from build123d import *

# Parameters (mm, degrees)
SKETCH1_R               = 11.7
BOSS_EXTRUDE1_DEPTH     = 35
SKETCH2_R               = 10
BOSS_EXTRUDE3_DEPTH     = 51.8
SKETCH3_R               = 3
CUT_EXTRUDE1_DEPTH      = 1
CUT_EXTRUDE1_DEPTH_BACK = 57.8
SKETCH6_W               = 28.4
SKETCH6_H               = 118.8
CUT_EXTRUDE3_DEPTH      = 36
SKETCH8_R               = 10
SKETCH8_R_2             = 3
CUT_EXTRUDE4_DEPTH      = 5
SKETCH7_R               = 4
SKETCH7_R_2             = 3
CUT_EXTRUDE5_DEPTH      = 5
FILLET1_R               = 10


with BuildPart() as part:
    # Sketch1 → Boss-Extrude1 (new body)
    with BuildSketch(Plane(origin=(0, 0, 0), x_dir=(0, 0, -1), z_dir=(1, 0, 0))):
        Polygon((-28.4, -59.4), (-23.4, -59.4), (-23.4, -14.4), (23.4, -14.4), (23.4, -59.4), (28.4, -59.4), (28.4, 59.4), (-28.4, 59.4), align=None)
        with Locations((0, 24)):
            Circle(SKETCH1_R, mode=Mode.SUBTRACT)
    extrude(amount=BOSS_EXTRUDE1_DEPTH)

    # Sketch2 → Boss-Extrude3 (add)
    with BuildSketch(Plane.XY.offset(28.4)):
        with Locations((17.5, -34.4)):
            Circle(SKETCH2_R)
        with BuildLine():
            Line((0, -24.717541634), (0, -13.4))
            Line((0, -13.4), (35, -13.4))
            Line((35, -13.4), (35, -24.717541634))
            ThreePointArc((35, -24.717541634), (17.5, -14.4), (0, -24.717541634))
        make_face()
    extrude(amount=-BOSS_EXTRUDE3_DEPTH)

    # Sketch3 → Cut-Extrude1 (cut, two sides)
    with BuildSketch(Plane.XY.offset(28.4)) as cut_extrude1_sk:
        with Locations((10.25, 49.4)):
            Circle(SKETCH3_R)
        with Locations((17.5, -34.4)):
            Circle(SKETCH3_R)
        with Locations((10.25, 2.3)):
            Circle(SKETCH3_R)
        with Locations((24.75, 2.3)):
            Circle(SKETCH3_R)
        with Locations((24.75, 49.4)):
            Circle(SKETCH3_R)
    extrude(amount=CUT_EXTRUDE1_DEPTH, mode=Mode.SUBTRACT)
    extrude(cut_extrude1_sk.sketch, amount=-CUT_EXTRUDE1_DEPTH_BACK, mode=Mode.SUBTRACT)

    # Sketch6 → Cut-Extrude3 (cut, through all)
    with BuildSketch(Plane(origin=(35, 0, 0), x_dir=(0, 0, -1), z_dir=(1, 0, 0))):
        with Locations((14.2, 0)):
            Rectangle(SKETCH6_W, SKETCH6_H)
    extrude(amount=-CUT_EXTRUDE3_DEPTH, mode=Mode.SUBTRACT)

    # Sketch8 → Cut-Extrude4 (cut)
    with BuildSketch(Plane(origin=(0, 0, 0), x_dir=(-1, 0, 0), z_dir=(0, 0, -1))):
        with Locations((-17.5, -34.4)):
            Circle(SKETCH8_R)
        with Locations((-17.5, -34.4)):
            Circle(SKETCH8_R_2, mode=Mode.SUBTRACT)
    extrude(amount=-CUT_EXTRUDE4_DEPTH, mode=Mode.SUBTRACT)

    # Sketch7 → Cut-Extrude5 (cut)
    with BuildSketch(Plane(origin=(0, 0, 0), x_dir=(-1, 0, 0), z_dir=(0, 0, -1))):
        with Locations((-24.75, 49.4)):
            Circle(SKETCH7_R)
        with Locations((-24.75, 49.4)):
            Circle(SKETCH7_R_2, mode=Mode.SUBTRACT)
        with Locations((-10.25, 49.4)):
            Circle(SKETCH7_R)
        with Locations((-10.25, 49.4)):
            Circle(SKETCH7_R_2, mode=Mode.SUBTRACT)
        with Locations((-24.75, 2.3)):
            Circle(SKETCH7_R)
        with Locations((-24.75, 2.3)):
            Circle(SKETCH7_R_2, mode=Mode.SUBTRACT)
        with Locations((-10.25, 2.3)):
            Circle(SKETCH7_R)
        with Locations((-10.25, 2.3)):
            Circle(SKETCH7_R_2, mode=Mode.SUBTRACT)
    extrude(amount=-CUT_EXTRUDE5_DEPTH, mode=Mode.SUBTRACT)

    # Fillet1
    fillet1_edges = [part.edges().sort_by_distance(p)[0] for p in [
        (0, 59.4, 14.2),
        (35, 59.4, 14.2),
    ]]
    fillet(fillet1_edges, radius=FILLET1_R)


solid = part.part
Source: CAD feature listing. Evaluate the final solid. Frame: model axes, mm. A direction names the side the tool comes from. Give positions to 0.01 mm unless a question says otherwise; leave off trailing zeros. Write each loop counter-clockwise with the first axis right and the second up, starting at its lowest first coordinate (ties: lowest second). Pieces come first, ordered by that corner, then holes. Notation, with made-up numbers: M -22.75,11 L 36.25,11 A25 ccw 36.25,35 Z; hole C 69,1.5 d4. An arc over 180 degrees is marked long. Return JSON: item names as keys, results as strings. Group by question number.
1) Draft query along Y for faces 3 (the face through (11.117, 45.495, 2.465)), 4 (the face through (3.01, 56.55, 14.4)), 5 (the face through (18, 47, 0)), 6 (the face through (17, -59.4, 26)). Return one class per face: released by +Y, released by -Y, zero draft, split by the parting line, or undercut.
2) Ray query, L1, parallel to X at y = 2.3, z = 13.75; L2, parallel to Y at x = 10.25, z = 1.3; L3, parallel to Y at x = 10.25, z = 12.75. Return the intervals inside material, ascending.
3) Cut plane D-D, the plane y = -34.4. Output: boundary loops of the cut face in (x, z).
4) Cut plane B-B, the plane x = 17.5. Output: boundary loops of the cut face in (y, z), then the cut area to 3 significant figures.
5) Cut plane A-A, the plane y = 2.3. Output: boundary loops of the cut face in (x, z), then the cut area to 3 significant figures.
6) Cut plane C-C, the plane x = 23. Output: boundary loops of the cut face in (y, z).
7) First-contact query: pin 1 Ø7 at (x, y) = (10.25, 49.4) entering from -Z; pin 2 Ø4 at (x, z) = (31, 16.5) entering from -Y; pin 3 Ø4 at (x, y) = (16.5, 25.5) entering from -Z. Flat tips, straight axial feed; report the tip coordinate or a pass-through.
8) Set-up query: faces 1 (the face through (22.88, -25.97, 14.33)), 2 (the face through (17.255, 24.257, 11.697)). Return all of +Z, -Z, +X, -X, +Y, -Y with unobstructed straight access to the full face (end or side cutting, diameter ignored); none if empty.
Data:
{
 "1": {"face 3": "undercut", "face 4": "released by +Y", "face 5": "zero draft", "face 6": "released by -Y"},
 "2": {"L1": "x = 0 to 7.25, 13.25 to 21.75, 27.75 to 35", "L2": "y = -15.76 to -1.7, 6.3 to 12.37, 35.63 to 45.4, 53.4 to 59.4", "L3": "y = -41.29 to -27.51, -15.76 to -0.7, 5.3 to 46.4, 52.4 to 59.4"},
 "3": {"outline": "M 0,23.4 L 7.5,23.4 L 7.5,5 L 14.5,5 L 14.5,28.4 L 0,28.4 Z; M 20.5,5 L 27.5,5 L 27.5,23.4 L 35,23.4 L 35,28.4 L 20.5,28.4 Z"},
 "4": {"outline": "M -59.4,23.4 L -44.4,23.4 L -44.4,5 L -37.4,5 L -37.4,28.4 L -59.4,28.4 Z; M -31.4,5 L -24.4,5 L -24.4,23.4 L -14.4,23.4 L -14.4,0 L 12.3,0 A11.7 cw 35.7,0 L 59.4,0 L 59.4,28.4 L -31.4,28.4 Z", "area": "2,330 mm²"},
 "5": {"outline": "M 0,0 L 6.25,0 L 6.25,5 L 7.25,5 L 7.25,28.4 L 0,28.4 Z; M 13.25,5 L 14.25,5 L 14.25,0 L 20.75,0 L 20.75,5 L 21.75,5 L 21.75,28.4 L 13.25,28.4 Z; M 27.75,5 L 28.75,5 L 28.75,0 L 35,0 L 35,28.4 L 27.75,28.4 Z", "area": "633 mm²"},
 "6": {"outline": "M -59.4,23.4 L -42.75,23.4 L -42.75,5 L -26.05,5 L -26.05,23.4 L -15.17,23.4 L -15.17,0 L -1.3,0 L -1.3,5 L -0.14,5 L -0.14,28.4 L -59.4,28.4 Z; M 4.74,5 L 5.9,5 L 5.9,0 L 12.3,0 A11.7 cw 35.7,0 L 45.8,0 L 45.8,5 L 46.96,5 L 46.96,28.4 L 4.74,28.4 Z; M 51.84,5 L 53,5 L 53,0 L 59.4,0 L 59.4,28.4 L 51.84,28.4 Z"},
 "7": {"pin 1": "stops at z = 5", "pin 2": "stops at y = -21.76", "pin 3": "stops at z = 11.16"},
 "8": {"face 1": "-Z", "face 2": "-Z, +X, -X"}
}
